The listing builds one solid part. Answer for the finished solid, in the listing's coordinates (mm). A direction names the side the tool comes from. Coordinates: 2 decimals unless noted, no trailing zeros. Loops run counter-clockwise (first coordinate to the right, second up) from the corner with the lowest first, then second, coordinate; pieces in that order, holes last. Notation, with made-up numbers: M -5,8 L 31,8 A19 cw 31,20 Z; hole C 18.25,-0.5 d9. An arc over 180 degrees is marked long. Return JSON: item names as keys, results as strings. Group by question number.
1. The mould has two halves that part along Z. Classify faces 4 (the face through (9, -2, -21)), 5 (the face through (0, -4.762, -8)), 6 (the face through (8.618, -6.716, 20.784)): pulls with the +Z half, pulls with the -Z half, needs draft (parallel to the pull), parting line crosses it, or undercut.
2. Section D-D (z = -18.5) is taken. Write down the section's boundary in (x, y), then the cut area to 3 significant figures.
3. Which of the six approach directions +Z, -Z, +X, -X, +Y, -Y give full straight-line access (tool end or side, diameter ignored) to faces 1 (the face through (7, -8.725, 22)), 2 (the face through (-9, -2, -22)), 3 (the face through (-31.144, -10.335, 4.705))?
4. Section A-A (z = 10) is taken. Write down the section's boundary in (x, y), then the cut area to 3 significant figures.
5. Section C-C (x = -19) is taken. Write down the section's boundary in (y, z), then the cut area to 3 significant figures.
6. Straight lines are drawn through the part: L1, parallel to Y at x = -21.5, z = 10.5; L2, parallel to X at y = -0.25, z = 5.5; L3, parallel to Y at x = 5.5, z = 9.5. For each, find the intervals that lie inside material, in ascending order. Write a range as from..to.
7. Given P1, Ø4.5, axis at x = 0, z = -10, coming from the +Y side; P2, Ø8, axis at x = -14.5, z = -21.5, coming from the +Y side; P3, Ø1.6, axis at x = 8.66, z = 5, coming from the -Y side; P4, Ø18, axis at x = 0, z = 0, coming from the -Y side, each flat-ended and moving along its own axis, determine where each tip first touches the part or whether it passes through.
8. Section B-B (y = -6) is taken. Write down the section's boundary in (x, z), then the cut area to 3 significant figures.
```python
from build123d import *

# Parameters (mm, degrees)
SPINDLE_START                             = 4.7625
SKETCH6_R                                 = 22.5
SKETCH6_R_2                               = 6.35
SPINDLE_CENTER_DEPTH                      = 3.9624
LOWER_START                               = 8.7249
LOWER_FLANGE_DEPTH                        = 3.175
UPPER_FLANGE_DEPTH                        = 4.7625
F_6_32_TAPPED_HOLE1_D                     = 2.7051
CBORE_START                               = -11.8999
CBORE_FOR_6_SOCKET_HEAD_CAP_SCREW1_OUTL_R = 3.57251
CBORE_FOR_6_SOCKET_HEAD_CAP_SCREW1_DEPTH  = 3.175
F_6_32_TAPPED_HOLE3_D                     = 2.7051
F_6_32_TAPPED_HOLE3_DEPTH                 = 9.49
F_6_32_TAPPED_HOLE3_TIP                   = 0.81269403


# Read off the part's stored shape, not the designer's step: CBORE for #6 Socket Head Cap Screw1
with BuildPart() as part:
    # Sketch6 → Spindle Center (new body)
    with BuildSketch(Plane.XZ.offset(SPINDLE_START)):
        with Locations(Location((0, 0, 0), (0, 0, 90))):
            Circle(SKETCH6_R)
        with Locations(Location((0, 0, 0), (0, 0, 90))):
            Circle(SKETCH6_R_2, mode=Mode.SUBTRACT)
    extrude(amount=SPINDLE_CENTER_DEPTH)

    # Sketch6<3> → Lower Flange (add)
    with BuildSketch(Plane.XZ.offset(LOWER_START)):
        with BuildLine():
            Line((0, -32.5), (0, -22.5))
            ThreePointArc((0, -22.5), (-4.596966983, -22.025392041), (-9, -20.621590627))
            Line((-9, -20.621590627), (-9, -31.228992939))
            ThreePointArc((-9, -31.228992939), (-4.544652323, -32.180679534), (0, -32.5))
        make_face()
        with BuildLine():
            Line((-9, -31.228992939), (-9, -20.621590627))
            ThreePointArc((-9, -20.621590627), (-22.025392041, 4.596966983), (0, 22.5))
            Line((0, 22.5), (0, 32.5))
            ThreePointArc((0, 32.5), (-32.180679534, 4.544652323), (-9, -31.228992939))
        make_face()
        with BuildLine():
            ThreePointArc((22.5, 0), (18.824850597, -12.323757544), (9, -20.621590627))
            Line((9, -20.621590627), (9, -31.228992939))
            ThreePointArc((9, -31.228992939), (25.968731197, -19.541622246), (32.5, 0))
            ThreePointArc((32.5, 0), (22.980970389, 22.980970389), (0, 32.5))
            Line((0, 32.5), (0, 22.5))
            ThreePointArc((0, 22.5), (15.909902577, 15.909902577), (22.5, 0))
        make_face()
        with BuildLine():
            Line((9, -31.228992939), (9, -20.621590627))
            ThreePointArc((9, -20.621590627), (4.596966983, -22.025392041), (0, -22.5))
            Line((0, -22.5), (0, -32.5))
            ThreePointArc((0, -32.5), (4.544652323, -32.180679534), (9, -31.228992939))
        make_face()
        with BuildLine():
            ThreePointArc((15, 0), (13.416407865, -6.708203932), (9, -12))
            Line((9, -12), (9, -20.621590627))
            ThreePointArc((9, -20.621590627), (18.824850597, -12.323757544), (22.5, 0))
            ThreePointArc((22.5, 0), (15.909902577, 15.909902577), (0, 22.5))
            Line((0, 22.5), (0, 15))
            ThreePointArc((0, 15), (10.606601718, 10.606601718), (15, 0))
        make_face()
        with BuildLine():
            Line((9, -20.621590627), (9, -12))
            ThreePointArc((9, -12), (4.74341649, -14.230249471), (0, -15))
            Line((0, -15), (0, -22.5))
            ThreePointArc((0, -22.5), (4.596966983, -22.025392041), (9, -20.621590627))
        make_face()
        with BuildLine():
            Line((0, -22.5), (0, -15))
            ThreePointArc((0, -15), (-4.74341649, -14.230249471), (-9, -12))
            Line((-9, -12), (-9, -20.621590627))
            ThreePointArc((-9, -20.621590627), (-4.596966983, -22.025392041), (0, -22.5))
        make_face()
        with BuildLine():
            Line((-9, -20.621590627), (-9, -12))
            ThreePointArc((-9, -12), (-14.230249471, 4.74341649), (0, 15))
            Line((0, 15), (0, 22.5))
            ThreePointArc((0, 22.5), (-22.025392041, 4.596966983), (-9, -20.621590627))
        make_face()
    extrude(amount=LOWER_FLANGE_DEPTH)

    # Sketch6<4> → Upper Flange (add)
    with BuildSketch(Plane.XZ):
        with BuildLine():
            Line((9, -12), (9, -31.228992939))
            ThreePointArc((9, -31.228992939), (0, 32.5), (-9, -31.228992939))
            Line((-9, -31.228992939), (-9, -12))
            ThreePointArc((-9, -12), (0, 15), (9, -12))
        make_face()
    extrude(amount=UPPER_FLANGE_DEPTH)

    # #6-32 Tapped Hole1 (through all)
    with Locations(Plane(origin=(0, -8.7249, 10), x_dir=(0, 0, -1), z_dir=(0, -1, 0))):
        with Locations((0, 0), (15, -8.660254038), (15, 8.660254038), (5, -8.660254038), (20, 0), (5, 8.660254038)):
            Hole(F_6_32_TAPPED_HOLE1_D / 2)

    # CBORE for #6 Socket Head Cap Screw1 outl → CBORE for #6 Socket Head Cap Screw1 (cut)
    with BuildSketch(Plane(origin=(0, 0, 0), x_dir=(1, 0, 0), z_dir=(0, 1, 0)).offset(CBORE_START)):
        with Locations((-27.574617084, -4.862148975)):
            Circle(CBORE_FOR_6_SOCKET_HEAD_CAP_SCREW1_OUTL_R)
        with Locations((-27.574617084, 4.862148975)):
            Circle(CBORE_FOR_6_SOCKET_HEAD_CAP_SCREW1_OUTL_R)
    extrude(amount=CBORE_FOR_6_SOCKET_HEAD_CAP_SCREW1_DEPTH, mode=Mode.SUBTRACT)

    # #6-32 Tapped Hole3
    with Locations(Plane(origin=(-27.574617084, 0, 4.862148975), x_dir=(0, 0, 1), z_dir=(0, 1, 0))):
        with Locations((0, 0), (-9.72429795, 0)):
            Hole(F_6_32_TAPPED_HOLE3_D / 2, depth=F_6_32_TAPPED_HOLE3_DEPTH)
            with Locations((0, 0, -(F_6_32_TAPPED_HOLE3_DEPTH + F_6_32_TAPPED_HOLE3_TIP / 2))):  # 118° drill point
                Cone(0, F_6_32_TAPPED_HOLE3_D / 2, F_6_32_TAPPED_HOLE3_TIP, mode=Mode.SUBTRACT)


solid = part.part
```
Worked out:
{
 "1": {"face 4": "needs draft", "face 5": "undercut", "face 6": "parting line crosses it"},
 "2": {"outline": "M -26.72,-11.9 L 26.72,-11.9 L 26.72,-8.72 L 12.81,-8.72 L 12.81,-4.76 L 26.72,-4.76 L 26.72,0 L 9,0 L 9,-4.76 L -9,-4.76 L -9,0 L -26.72,0 L -26.72,-4.76 L -12.81,-4.76 L -12.81,-8.72 L -26.72,-8.72 Z", "area": "440 mm^2"},
 "3": {"face 1": "none", "face 2": "-Z, +Y", "face 3": "-Y"},
 "4": {"outline": "M -30.92,-11.9 L -11.18,-11.9 L -11.18,-8.72 L -1.35,-8.72 L -1.35,-4.76 L -11.18,-4.76 L -11.18,0 L -30.92,0 L -30.92,-4.76 L -20.16,-4.76 L -20.16,-8.72 L -30.92,-8.72 Z; M 1.35,-8.72 L 11.18,-8.72 L 11.18,-11.9 L 30.92,-11.9 L 30.92,-8.72 L 20.16,-8.72 L 20.16,-4.76 L 30.92,-4.76 L 30.92,0 L 11.18,0 L 11.18,-4.76 L 1.35,-4.76 Z", "area": "462 mm^2"},
 "5": {"outline": "M -11.9,-26.37 L -8.72,-26.37 L -8.72,-12.05 L -4.76,-12.05 L -4.76,-26.37 L 0,-26.37 L 0,26.37 L -4.76,26.37 L -4.76,12.05 L -8.72,12.05 L -8.72,26.37 L -11.9,26.37 Z", "area": "514 mm^2"},
 "6": {"L1": "-11.9..-8.72, -4.76..0", "L2": "-32.03..-28.77, -26.38..-13.96, 13.96..32.03", "L3": "-8.72..-4.76"},
 "7": {"P1": "y = -4.76", "P2": "y = 0", "P3": "through", "P4": "y = -8.72"},
 "8": {"outline": "C 0,0 d45; hole C -8.66,-5 d2.71; hole C -8.66,5 d2.71; hole C 0,0 d12.7; hole C 0,-10 d2.71; hole C 0,10 d2.71; hole C 8.66,-5 d2.71; hole C 8.66,5 d2.71", "area": "1,430 mm^2"}
}
